Source: CAD feature listing. Evaluate the final solid. Frame: model axes, mm. Give positions to 0.01 mm unless a question says otherwise; leave off trailing zeros. Loops run counter-clockwise (first coordinate to the right, second up) from the corner with the lowest first, then second, coordinate; pieces in that order, holes last. Notation, with made-up numbers: (2.5, -38.75) -> (38.5, -38.75) arc R31 cw to (38.5, -1.75) -> close; hole circle Ø8 at (-10, -6.5). An arc over 180 degrees is marked (long way). Put each result on its own line as item: value.
```python
from build123d import *

# Parameters (mm, degrees)
CROQUIS1_R              = 1.25
SALIENTE_EXTRUIR1_DEPTH = 3
CHAFL_N1_SIZE           = 1


with BuildPart() as part:
    # Croquis1 → Saliente-Extruir1 (new body)
    with BuildSketch(Plane(origin=(0, 0, 0), x_dir=(1, 0, 0), z_dir=(0, 1, 0))):
        with BuildLine():
            Line((-31.108771954, -40.5), (-30.108771954, -39.5))
            Line((-30.108771954, -39.5), (-30.108771954, -21.5))
            Line((-30.108771954, -21.5), (-5.108771954, -21.5))
            Line((-5.108771954, -21.5), (-5.108771954, -39.5))
            Line((-5.108771954, -39.5), (-4.108771954, -40.5))
            Line((-4.108771954, -40.5), (1, -40.5))
            ThreePointArc((1, -40.5), (2.414213562, -39.914213562), (3, -38.5))
            Line((3, -38.5), (3, 1))
            ThreePointArc((3, 1), (2.414213562, 2.414213562), (1, 3))
            Line((1, 3), (-4.108771954, 3))
            Line((-4.108771954, 3), (-5.108771954, 2))
            Line((-5.108771954, 2), (-5.108771954, -11))
            Line((-5.108771954, -11), (-6.108771954, -12))
            Line((-6.108771954, -12), (-29.108771954, -12))
            Line((-29.108771954, -12), (-30.108771954, -11))
            Line((-30.108771954, -11), (-30.108771954, 2))
            Line((-30.108771954, 2), (-31.108771954, 3))
            Line((-31.108771954, 3), (-38.5, 3))
            ThreePointArc((-38.5, 3), (-39.914213562, 2.414213562), (-40.5, 1))
            Line((-40.5, 1), (-40.5, -38.5))
            ThreePointArc((-40.5, -38.5), (-39.914213562, -39.914213562), (-38.5, -40.5))
            Line((-38.5, -40.5), (-31.108771954, -40.5))
        make_face()
        with Locations((-37.5, -37.5)):
            Circle(CROQUIS1_R, mode=Mode.SUBTRACT)
        with Locations((-37.5, 0)):
            Circle(CROQUIS1_R, mode=Mode.SUBTRACT)
        with Locations((0, -37.5)):
            Circle(CROQUIS1_R, mode=Mode.SUBTRACT)
        Circle(CROQUIS1_R, mode=Mode.SUBTRACT)
    extrude(amount=SALIENTE_EXTRUIR1_DEPTH)

    # Chaflán1
    chafl_n1_edges = [part.edges().sort_by_distance(p)[0] for p in [
        (-4.608771954, 0, 40),
        (-30.608771954, 0, 40),
        (-4.608771954, 0, -2.5),
        (-5.108771954, 3, 4.5),
        (-30.608771954, 0, -2.5),
        (-5.608771954, 0, 11.5),
        (-30.108771954, 0, 4.5),
        (-29.608771954, 0, 11.5),
        (-17.608771954, 0, 12),
        (-5.108771954, 0, 30.5),
        (-30.108771954, 0, 30.5),
        (-5.108771954, 1.5, 21.5),
        (-17.608771954, 0, 21.5),
        (-30.108771954, 1.5, 21.5),
    ]]
    chamfer(chafl_n1_edges, length=CHAFL_N1_SIZE)


solid = part.part
```
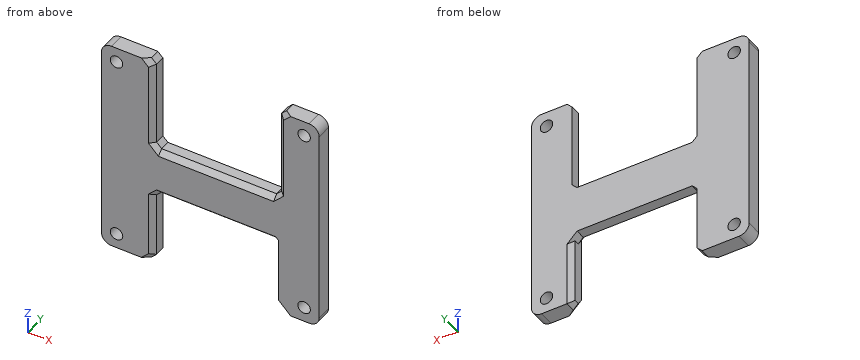
(1) Section D-D on y = 0.5. Return loops of the section in (x, z), then the cut area to 3 significant figures.
Calculated:
outline: (-40.5, -1) arc R2 ccw to (-38.5, -3) -> (-31.82, -3) -> (-30.61, -1.79) -> (-30.61, 11.21) -> (-29.32, 12.5) -> (-5.9, 12.5) -> (-5.11, 11.71) -> (-5.11, -1.29) -> (-3.4, -3) -> (1, -3) arc R2 ccw to (3, -1) -> (3, 38.5) arc R2 ccw to (1, 40.5) -> (-3.4, 40.5) -> (-4.61, 39.29) -> (-4.61, 22.5) -> (-6.11, 21) -> (-29.11, 21) -> (-30.61, 22.5) -> (-30.61, 39.29) -> (-31.82, 40.5) -> (-38.5, 40.5) arc R2 ccw to (-40.5, 38.5) -> close; hole circle Ø2.5 at (-37.5, 0); hole circle Ø2.5 at (-37.5, 37.5); hole circle Ø2.5 at (0, 0); hole circle Ø2.5 at (0, 37.5)
area: 967 mm²
(2) Line query: probe 1 along Z at (x, y) = (0, 2); probe 2 along X at (y, z) = (1.25, 0); probe 3 along X at (y, z) = (0.75, 37.5). Output: solid intervals per line, ascending. Write a range as from..to.
Calculated:
probe 1: z = -3..-1.25, 1.25..36.25, 38.75..40.5
probe 2: x = -40.5..-38.75, -36.25..-30.11, -5.11..-1.25, 1.25..3
probe 3: x = -40.5..-38.75, -36.25..-30.36, -4.86..-1.25, 1.25..3
(3) Section A-A on x = -37.5. Return loops of the section in (y, z), then the cut area to 4 significant figures.
Calculated:
outline: (0, -3) -> (3, -3) -> (3, -1.25) -> (0, -1.25) -> close; (0, 1.25) -> (3, 1.25) -> (3, 36.25) -> (0, 36.25) -> close; (0, 38.75) -> (3, 38.75) -> (3, 40.5) -> (0, 40.5) -> close
area: 115.5 mm²
(4) First-contact query: P1, Ø10, axis at x = -16, z = 7.5, coming from the -Y side; P2, Ø8, axis at x = -9, z = 28, coming from the -Y side; P3, Ø1, axis at x = -20.5, y = 2, coming from the +Z side. Flat tips, straight axial feed; report the tip coordinate or a pass-through.
Calculated:
P1: stops at y = 0.5
P2: stops at y = 0.89
P3: stops at z = 21.5
(5) Section B-B on z = 37.5. Return loops of the section in (x, y), then the cut area to 3 significant figures.
Calculated:
outline: (-40.5, 0) -> (-38.75, 0) -> (-38.75, 3) -> (-40.5, 3) -> close; (-36.25, 0) -> (-31.11, 0) -> (-30.11, 1) -> (-30.11, 3) -> (-36.25, 3) -> close; (-5.11, 1) -> (-4.11, 0) -> (-1.25, 0) -> (-1.25, 3) -> (-5.11, 3) -> close; (1.25, 0) -> (3, 0) -> (3, 3) -> (1.25, 3) -> close
area: 39.5 mm²
(6) Section C-C on z = 6. Return loops of the section in (x, y).
Calculated:
outline: (-40.5, 0) -> (-31.11, 0) -> (-30.11, 1) -> (-30.11, 3) -> (-40.5, 3) -> close; (-5.11, 0) -> (3, 0) -> (3, 3) -> (-4.11, 3) -> (-5.11, 2) -> close
